Here's the drawing with two shaded views (mm, measured from the low corner). I have some questions. Coordinates: 2 decimals unless noted, no trailing zeros. Write each loop counter-clockwise with the first axis right and the second up, starting at its lowest first coordinate (ties: lowest second). Pieces come first, ordered by that corner, then holes.
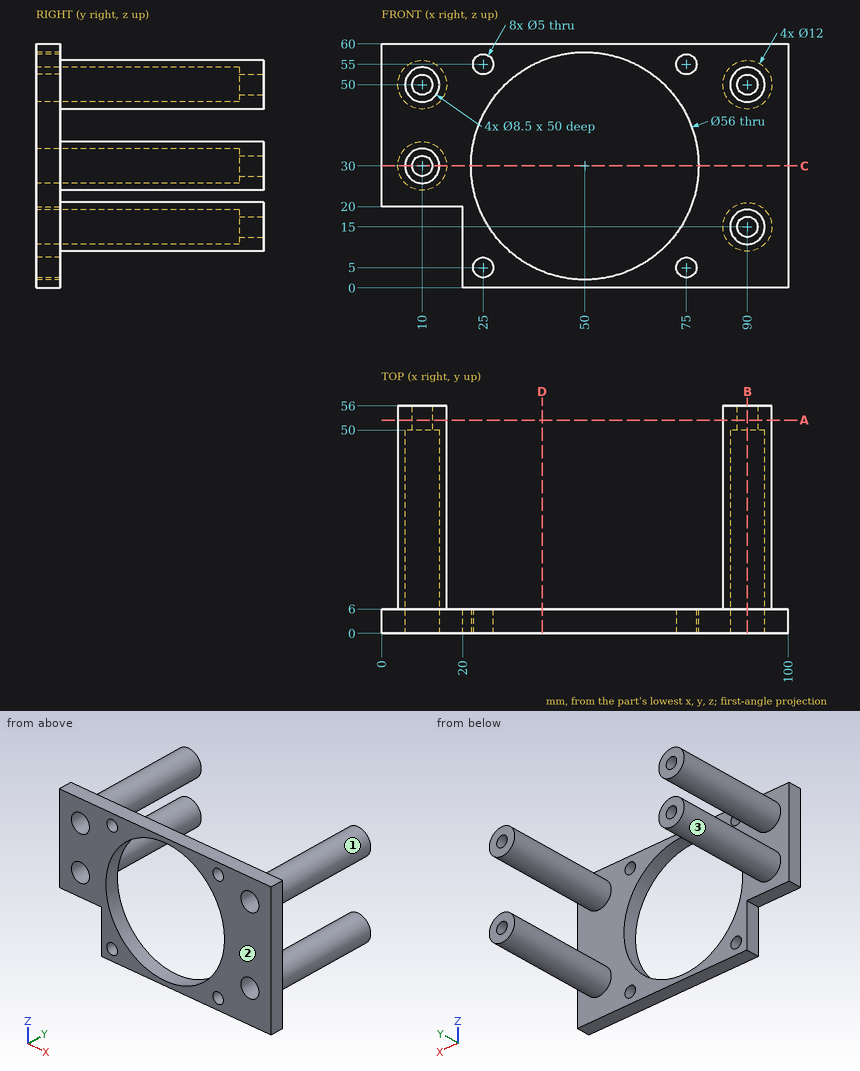
Item 1: I want a section at C-C, the plane z = 30. List the corners of the cut face in (x, y) for me, then the cut area to 3 significant figures.
Item 2: I want a section at A-A, the plane y = 52.5. List the corners of the cut face in (x, z) for me.
Item 3: Will these pins go through, and if not, where does the flat tip stop? pin 1 Ø12 at (y, z) = (28, 21) entering from -X; pin 2 Ø7 at (x, z) = (88, 13.5) entering from -Y; pin 3 Ø6.5 at (x, z) = (25, 55) entering from +Y; pin 4 Ø1.8 at (y, z) = (4.5, 10) entering from -X.
Item 4: If we mould it in two halves opening along Z, with no side actions, what happens to the marked faces 1, 2 and 3? For each: released by +Z, released by -Z, zero draft, split by the parting line, or undercut.
Item 5: I want a section at D-D, the plane x = 39.5. List the corners of the cut face in (y, z) for me, then the cut area to 3 significant figures.
Item 6: I want a section at B-B, the plane x = 90. List the corners of the cut face in (y, z) for me, then the cut area to 3 significant figures.
Item 7: If I drill on line 1 along Z through (x, y) = (10, 54); line 2 along Z through (x, y) = (90, 33.5); line 3 along X through (y, z) = (51, 30), over which ranges is the centre line in solid material (lowest first)?
Taken from the geometry:
1. outline: (0, 0) - (5.75, 0) - (5.75, 50) - (7.5, 50) - (7.5, 56) - (4, 56) - (4, 6) - (0, 6) - close; (12.5, 50) - (14.25, 50) - (14.25, 0) - (22, 0) - (22, 6) - (16, 6) - (16, 56) - (12.5, 56) - close; (78, 0) - (100, 0) - (100, 6) - (78, 6) - close
1. area: 409 mm2
2. outline: circle Ø12 at (10, 30); circle Ø12 at (10, 50); circle Ø12 at (90, 15); circle Ø12 at (90, 50); hole circle Ø5 at (10, 30); hole circle Ø5 at (10, 50); hole circle Ø5 at (90, 15); hole circle Ø5 at (90, 50)
3. pin 1: stops at x = 4.8
3. pin 2: stops at y = 0
3. pin 3: stops at y = 6
3. pin 4: stops at x = 20
4. face 1: undercut
4. face 2: zero draft
4. face 3: undercut
5. outline: (0, 0) - (6, 0) - (6, 4.04) - (0, 4.04) - close; (0, 55.96) - (6, 55.96) - (6, 60) - (0, 60) - close
5. area: 48.5 mm2
6. outline: (0, 0) - (6, 0) - (6, 9) - (56, 9) - (56, 12.5) - (50, 12.5) - (50, 10.75) - (0, 10.75) - close; (0, 19.25) - (50, 19.25) - (50, 17.5) - (56, 17.5) - (56, 21) - (6, 21) - (6, 44) - (56, 44) - (56, 47.5) - (50, 47.5) - (50, 45.75) - (0, 45.75) - close; (0, 54.25) - (50, 54.25) - (50, 52.5) - (56, 52.5) - (56, 56) - (6, 56) - (6, 60) - (0, 60) - close
6. area: 650 mm2
7. line 1: z = 24 to 27.5, 32.5 to 36, 44 to 47.5, 52.5 to 56
7. line 2: z = 9 to 10.75, 19.25 to 21, 44 to 45.75, 54.25 to 56
7. line 3: x = 4 to 7.5, 12.5 to 16
